Check sheet for the modelled part. Datum: model origin and axes. Units: mm. A direction names the side the tool comes from. Round coordinates to 2 decimals unless told otherwise and drop trailing zeros. Order: outer loops, then holes, each group sorted by start corner. A loop starts at its lowest first (then second) coordinate and runs counter-clockwise, first axis right, second up.
(1) Sectioned sample at C-C, the plane y = -1. Enter the section's corners in (x, z).
(2) Sectioned sample at B-B, the plane z = 5.5. Enter the section's corners in (x, y).
(3) Depth check by flat-ended pin: pin 1 (2 mm diameter, centred on x = 0, y = 0, fed in from -Z). Enter the tip coordinate at first touch or a pass-through.
(4) Thickness scan on probe 1 along X at (y, z) = (0, 3.5); probe 2 along X at (y, z) = (1, 6.5); probe 3 along Y at (x, z) = (-0.75, 1.5). Record the ranges inside material, lowest first.
(5) Sectioned sample at A-A, the plane x = 0. Enter the section's corners in (y, z).
(6) Sectioned sample at D-D, the plane y = -3.5. Enter the section's corners in (x, z), and give its area (3 significant figures).
(7) Tool access check on faces 1 (the cylindrical face through (0, -4, 6)), 2 (the cylindrical face through (-0.27, -1.22, 6.07)). Record the directions out of +Z, -Z, +X, -X, +Y, -Y that give a thin tool (end or side, any length) a straight path to the whole face; none if there is none.
(8) Mould release check, pull along Y, two halves, no side actions. Record for faces 3 (the flat face through (0, 0, 0)), 4 (the cylindrical face through (0, 4, 6)), 5 (the flat face through (0, 0, 0.3)): released by +Y, released by -Y, zero draft, split by the parting line, or undercut.
```python
from build123d import *

# Parameters (mm, degrees)
SKETCH1_R           = 1.25
BOSS_EXTRUDE1_DEPTH = 12
SKETCH3_R           = 1.25
BOSS_EXTRUDE2_DEPTH = 0.3


with BuildPart() as part:
    # Sketch1 → Boss-Extrude1 (new body)
    with BuildSketch(Plane.XY):
        with BuildLine():
            Line((3.5, 1.936491673), (3.5, -1.936491673))
            ThreePointArc((3.5, -1.936491673), (0, -4), (-3.5, -1.936491673))
            Line((-3.5, -1.936491673), (-3.5, 1.936491673))
            ThreePointArc((-3.5, 1.936491673), (0, 4), (3.5, 1.936491673))
        make_face()
        Circle(SKETCH1_R, mode=Mode.SUBTRACT)
    extrude(amount=BOSS_EXTRUDE1_DEPTH)

    # Sketch3 → Boss-Extrude2 (add)
    with BuildSketch(Plane(origin=(0, 0, 0), x_dir=(-1, 0, 0), z_dir=(0, 0, -1))):
        Circle(SKETCH3_R)
    extrude(amount=-BOSS_EXTRUDE2_DEPTH)


solid = part.part
```
Derived:
1. outline: (-3.5, 0) - (3.5, 0) - (3.5, 12) - (0.75, 12) - (0.75, 0.3) - (-0.75, 0.3) - (-0.75, 12) - (-3.5, 12) - close
2. outline: (-3.5, -1.94) arc R4 ccw to (3.5, -1.94) - (3.5, 1.94) arc R4 ccw to (-3.5, 1.94) - close; hole circle Ø2.5 at (0, 0)
3. pin 1: stops at z = 0
4. probe 1: x = -3.5 to -1.25, 1.25 to 3.5
4. probe 2: x = -3.5 to -0.75, 0.75 to 3.5
4. probe 3: y = -3.93 to -1, 1 to 3.93
5. outline: (-4, 0) - (4, 0) - (4, 12) - (1.25, 12) - (1.25, 0.3) - (-1.25, 0.3) - (-1.25, 12) - (-4, 12) - close
6. outline: (-1.94, 0) - (1.94, 0) - (1.94, 12) - (-1.94, 12) - close
6. area: 46.5 mm2
7. face 1: +Z, -Z, -Y
7. face 2: +Z
8. face 3: zero draft
8. face 4: released by +Y
8. face 5: undercut
